Verification items for the finished model (mm, model axes). A direction names the side the tool comes from. Give positions to 0.01 mm unless a question says otherwise; leave off trailing zeros. Write each loop counter-clockwise with the first axis right and the second up, starting at its lowest first coordinate (ties: lowest second). Pieces come first, ordered by that corner, then holes. Notation, with made-up numbers: M 35,56.5 L 67,56.5 A29 cw 67,95.5 Z; hole C 57,26.25 d10. An arc over 180 degrees is marked long. Write item = value, one per line.
from build123d import *

# Parameters (mm, degrees)
F1_DEPTH = 4.7625
F2_R     = 2
F3_DEPTH = 50
F4_R     = 3.5
F4_R_2   = 2
F5_DEPTH = 40
F6_R     = 2
F7_DEPTH = 15.1971524227
F8_R     = 2
F9_DEPTH = 70.1490577065


# Not quite as in the source:
# - a length typed as a fraction of an inch, garbled in the dataset ("3 / 203.2 mm" for 3/8 in), is restored


with BuildPart() as f1:
    # F0 (on Right) → F1 (new body, symmetric)
    with BuildSketch(Plane.YZ):
        Polygon((0.8673048454, 75.500738686), (-9.525, 69.500738686), (-9.525, 14.4948291982), (-0.8673048454, -0.500738686), (9.525, 5.499261314), (9.525, 60.5051708018), align=None)
    extrude(amount=F1_DEPTH, both=True)

    # F2 (on face) → F3 (join)
    with BuildSketch(Plane(origin=(0, 0, 0), x_dir=(1, 0, 0), z_dir=(0, 0.5, -0.8660254038))):
        with Locations((0, -4.9985226281)):
            Circle(F2_R)
    extrude(amount=-F3_DEPTH)

    # F4 (on face) → F5 (cut)
    with BuildSketch(Plane(origin=(0, -25, 43.3012701892), x_dir=(1, 0, 0), z_dir=(0, -0.5, 0.8660254038))):
        with Locations((0, 4.9985226281)):
            Circle(F4_R)
        with Locations((0, 4.9985226281)):
            Circle(F4_R_2, mode=Mode.SUBTRACT)
        with Locations((0, 4.9985226281)):
            Circle(F4_R_2)
    extrude(amount=-F5_DEPTH, mode=Mode.SUBTRACT)

    # F6 (on face) → F7 (cut, through all)
    with BuildSketch(Plane(origin=(0, -5, 8.6602540378), x_dir=(1, 0, 0), z_dir=(0, -0.5, 0.8660254038))):
        with Locations((0, 4.9985226281)):
            Circle(F6_R)
    extrude(amount=-F7_DEPTH, mode=Mode.SUBTRACT)

    # F8 (on face) → F9 (cut, through all)
    with BuildSketch(Plane(origin=(0, -32.4759526419, 56.25), x_dir=(1, 0, 0), z_dir=(0, -0.5, 0.8660254038))):
        with Locations((0, 32.5014773719)):
            Circle(F8_R)
    extrude(amount=-F9_DEPTH, mode=Mode.SUBTRACT)


solid = f1.part
1) Cross-section at A-A on x = -0.25. Record the boundary of the cut face in (y, z) (1 decimal).
From the geometry:
outline = M -9.5,14.5 L -0.9,-0.5 L 2.6,1.5 L -2.4,10.2 L -3.7,9.4 L -9.5,19.5 Z; M -9.5,33.5 L 2.4,12.9 L 1,12.2 L 6,3.5 L 9.5,5.5 L 9.5,44.5 L -6,71.5 L -9.5,69.5 Z; M -2.6,73.5 L 9.5,52.5 L 9.5,60.5 L 0.9,75.5 Z
2) Material ranges on probe 1 along Z at (x, y) = (0.5, -1); probe 2 along Z at (x, y) = (-0.75, -5); probe 3 along Y at (x, z) = (0.75, 18.5) (3 decimals), recorded low to high. Write a range as from..to.
From the geometry:
probe_1 = -0.27..7.86, 18.66..62.86, 70.61..74.42
probe_2 = 6.66..11.82, 25.49..69.96
probe_3 = -9.525..-8.857, -0.962..9.525
3) Depth check by flat-ended pin: P1, Ø4, axis at x = -0.5, y = 7, coming from the -Z side; P2, Ø4, axis at x = -4, z = 65, coming from the +Y side; P3, Ø3, axis at x = -2, y = 5, coming from the +Z side. Enter the tip coordinate at first touch or a pass-through.
From the geometry:
P1 = 3.09
P2 = 8.08
P3 = 70.94
4) Draft check along X on faces 3 (the flat face through (-4.762, 0, 38)), 4 (the cylindrical face through (-0.43, 1.66, 58.22)), 5 (the flat face through (2.18, 4.26, 2.46)). Enter one of: +X half, -X half, draft (parallel to the pull), parting line (faces both ways), or undercut.
From the geometry:
face_3 = -X half
face_4 = undercut
face_5 = draft
5) Tool access check on faces 1 (the flat face through (0, -9.525, 42)), 2 (the flat face through (-0.049, -2.649, 10.017)). Record the directions out of +Z, -Z, +X, -X, +Y, -Y that give a thin tool (end or side, any length) a straight path to the whole face; none if there is none.
From the geometry:
face_1 = +Z, -Z, +X, -X, -Y
face_2 = none
